```python
from build123d import *

# Parameters (mm, degrees)
SKETCH1_R           = 1.75
SKETCH1_R_2         = 3.45
BOSS_EXTRUDE1_DEPTH = 2


with BuildPart() as part:
    # Sketch1 → Boss-Extrude1 (new body)
    with BuildSketch(Plane.XY):
        with BuildLine():
            Line((-3.545417743, 13.027011553), (-4.176634672, 6.056009592))
            ThreePointArc((-4.176634672, 6.056009592), (-4.493207513, 4.516501974), (-5.145282945, 3.086432151))
            ThreePointArc((-5.145282945, 3.086432151), (0, -6), (5.145282945, 3.086432151))
            ThreePointArc((5.145282945, 3.086432151), (4.493207513, 4.516501974), (4.176634672, 6.056009592))
            Line((4.176634672, 6.056009592), (3.545417743, 13.027011553))
            ThreePointArc((3.545417743, 13.027011553), (3.608859175, 14.389566924), (4.038179283, 15.684273917))
            ThreePointArc((4.038179283, 15.684273917), (0, 22.17), (-4.038179283, 15.684273917))
            ThreePointArc((-4.038179283, 15.684273917), (-3.608859175, 14.389566924), (-3.545417743, 13.027011553))
        make_face()
        with Locations((0, 17.67)):
            Circle(SKETCH1_R, mode=Mode.SUBTRACT)
        Circle(SKETCH1_R_2, mode=Mode.SUBTRACT)
    extrude(amount=BOSS_EXTRUDE1_DEPTH)


solid = part.part
```
Read the model definition and answer for the solid it produces. Units are mm, in the model's axes. A direction names the side the tool comes from. Coordinates: 2 decimals unless noted, no trailing zeros. Order: outer loops, then holes, each group sorted by start corner. A loop starts at its lowest first (then second) coordinate and runs counter-clockwise, first axis right, second up. Notation, with made-up numbers: (-27, -32) - (13, -32) arc R21 cw to (13, -12) - close; hole circle Ø7 at (15.5, -7). An arc over 180 degrees is marked (long way). Answer as a JSON object with one key per item and string values. Group by question number.
Item 1: Section C-C (x = -2) is taken. Give the vertices of the cut face in (y, z), plus the area to 3 significant figures.
Item 2: Section A-A (y = -3) is taken. Give the vertices of the cut face in (x, z).
Item 3: A flat-ended cylindrical pin translates along its axis: P1, Ø1, axis at x = -1.5, z = 0.5, coming from the -Y side. Find the tip coordinate at first contact, or state that the pin passes through.
Item 4: Consider probe 1 along Y at (x, z) = (1, 1.2); probe 2 along X at (y, z) = (16.75, 1.45); probe 3 along X at (y, z) = (19.25, 0.85). Determine where each line is inside the solid, lowest interval first. Write a range as from..to.
Item 5: Section D-D (z = 1.65) is taken. Give the vertices of the cut face in (x, y), plus the area to 3 significant figures.
Item 6: Section B-B (x = 0) is taken. Give the vertices of the cut face in (y, z), plus the area to 3 significant figures.
Item 7: The mould has two halves that part along Y. Classify faces 1 (the face through (0, -6, 1)), 2 (the face through (0, 8, 2)), 3 (the face through (4.5, 4.5, 1)): +Y half, -Y half, draft (parallel to the pull), parting line (faces both ways), or undercut.
Item 8: A tool of negligible diameter and unlimited length cuts with its end or side. For faces 4 (the face through (-4.5, 4.5, 1)), 5 (the face through (3.865, 9.493, 0.986)), 6 (the face through (0, 8, 0)), from which of +Z, -Z, +X, -X, +Y, -Y can it reach the whole face along a straight path? Write none if from no direction.
Results are:
{
 "1": {"outline": "(-5.66, 0) - (-2.81, 0) - (-2.81, 2) - (-5.66, 2) - close; (2.81, 0) - (21.7, 0) - (21.7, 2) - (2.81, 2) - close", "area": "43.5 mm^2"},
 "2": {"outline": "(-5.2, 0) - (-1.7, 0) - (-1.7, 2) - (-5.2, 2) - close; (1.7, 0) - (5.2, 0) - (5.2, 2) - (1.7, 2) - close"},
 "3": {"P1": "stops at y = -5.92"},
 "4": {"probe 1": "y = -5.92..-3.3, 3.3..16.23, 19.11..22.06", "probe 2": "x = -4.4..-1.49, 1.49..4.4", "probe 3": "x = -4.21..-0.75, 0.75..4.21"},
 "5": {"outline": "(-5.15, 3.09) arc R6 ccw (long way) to (5.15, 3.09) arc R7 cw to (4.18, 6.06) - (3.55, 13.03) arc R5 cw to (4.04, 15.68) arc R4.5 ccw (long way) to (-4.04, 15.68) arc R5 cw to (-3.55, 13.03) - (-4.18, 6.06) arc R7 cw to start; hole circle Ø6.9 at (0, 0); hole circle Ø3.5 at (0, 17.67)", "area": "194 mm^2"},
 "6": {"outline": "(-6, 0) - (-3.45, 0) - (-3.45, 2) - (-6, 2) - close; (3.45, 0) - (15.92, 0) - (15.92, 2) - (3.45, 2) - close; (19.42, 0) - (22.17, 0) - (22.17, 2) - (19.42, 2) - close", "area": "35.5 mm^2"},
 "7": {"face 1": "parting line", "face 2": "draft", "face 3": "undercut"},
 "8": {"face 4": "+Z, -Z, -X", "face 5": "+Z, -Z, +X", "face 6": "-Z, +X, -X, +Y, -Y"}
}
